Model file for the job. Use its own axes, mm. A direction names the side the tool comes from. Round coordinates to 2 decimals unless told otherwise and drop trailing zeros. Loops run counter-clockwise (first coordinate to the right, second up) from the corner with the lowest first, then second, coordinate; pieces in that order, holes last. Notation, with made-up numbers: M 6,-7.75 L 48,-7.75 A18 cw 48,-3.75 Z; hole C 30.5,-24 d10. An arc over 180 degrees is marked long. Use a Markdown table: item, result. Add a question column.
Item 1: Two-plate mould, pull along Y, no slides. Class faces 4 (the flat face through (8, -1, 3.6)), 5 (the cylindrical face through (-2.8, 0.1, 3.8)), 6 (the cylindrical face through (-2.15, 0.09, 3.69)): +Y half, -Y half, draft (parallel to the pull), parting line (faces both ways), or undercut.
Item 2: Saw through at C-C on z = 3.1. Write the cut outline in (x, y) (3 decimals), then the cut area to 3 significant figures.
Item 3: Wall check: L1, parallel to Y at x = 0, z = 3.1 (3 decimals); L2, parallel to Z at x = 3.5, y = 2.55; L3, parallel to Z at x = -0.75, y = -0.25. Give the ranges that are in metal, low to high. Write a range as from..to.
Item 4: Saw through at B-B on x = 11. Write the cut outline in (y, z).
Item 5: Saw through at D-D on x = 8. Write the cut outline in (y, z).
Item 6: Pin check, flat tips, straight feed: P1, Ø2, axis at y = 0.5, z = 1, coming from the -X side; P2, Ø2, axis at x = 0, y = 0, coming from the -Z side; P3, Ø2, axis at x = 0, y = 0.5, coming from the +Z side; P4, Ø1.5, axis at x = 9.5, z = 2.5, coming from the +Y side. Stop position of each tip, or through.
Item 7: Tool access for faces 1 (the cylindrical face through (-3, 0, 1)), 2 (the flat face through (-1, 0, 3.3)), 3 (the cylindrical face through (4.6, -0.3, 2.6)): list every direction of +Z, -Z, +X, -X, +Y, -Y with a clear straight run to the whole face (end or side of a thin tool).
```python
from build123d import *

# Parameters (mm, degrees)
SKETCH2_R           = 3
SKETCH2_R_2         = 2.8
BOSS_EXTRUDE1_DEPTH = 3.6
SKETCH2_3_R         = 2.8
SKETCH2_3_R_2       = 2.15
BOSS_EXTRUDE2_DEPTH = 4.1
BOSS_EXTRUDE3_START = 2.7
SKETCH2_4_R         = 2.15
SKETCH2_4_R_2       = 0.625
BOSS_EXTRUDE3_DEPTH = 0.6
SKETCH2_5_R         = 2.15
BOSS_EXTRUDE4_DEPTH = 2.7
BOSS_EXTRUDE5_START = 3.6
SKETCH2_6_R         = 0.5
BOSS_EXTRUDE5_DEPTH = 2


with BuildPart() as part:
    # Sketch2 → Boss-Extrude1 (new body)
    with BuildSketch(Plane.XY):
        Circle(SKETCH2_R)
        Circle(SKETCH2_R_2, mode=Mode.SUBTRACT)
    extrude(amount=BOSS_EXTRUDE1_DEPTH)

    # Sketch2<3> → Boss-Extrude2 (add)
    with BuildSketch(Plane.XY):
        Circle(SKETCH2_3_R)
        Circle(SKETCH2_3_R_2, mode=Mode.SUBTRACT)
    extrude(amount=BOSS_EXTRUDE2_DEPTH)

    # Sketch2<4> → Boss-Extrude3 (add)
    with BuildSketch(Plane.XY.offset(BOSS_EXTRUDE3_START)):
        Circle(SKETCH2_4_R)
        Circle(SKETCH2_4_R_2, mode=Mode.SUBTRACT)
    extrude(amount=BOSS_EXTRUDE3_DEPTH)

    # Sketch2<5> → Boss-Extrude4 (add)
    with BuildSketch(Plane.XY):
        Circle(SKETCH2_5_R)
        Polygon((-0.374241043, 1.760665681), (0, 2), (0.374241043, 1.760665681), (0.813473286, 1.827090915), (1.058013454, 1.45623059), (1.486289651, 1.338261213), (1.558845727, 0.9), (1.902113033, 0.618033989), (1.790139412, 0.188151234), (1.989043791, -0.209056927), (1.711901729, -0.55623059), (1.732050808, -1), (1.337660686, -1.204435091), (1.175570505, -1.618033989), (0.732125958, -1.644381824), (0.415823382, -1.956295201), (0, -1.8), (-0.415823382, -1.956295201), (-0.732125958, -1.644381824), (-1.175570505, -1.618033989), (-1.337660686, -1.204435091), (-1.732050808, -1), (-1.711901729, -0.55623059), (-1.989043791, -0.209056927), (-1.790139412, 0.188151234), (-1.902113033, 0.618033989), (-1.558845727, 0.9), (-1.486289651, 1.338261213), (-1.058013454, 1.45623059), (-0.813473286, 1.827090915), align=None, mode=Mode.SUBTRACT)
    extrude(amount=BOSS_EXTRUDE4_DEPTH)

    # Sketch2<6> → Boss-Extrude5 (add)
    with BuildSketch(Plane.XY.offset(BOSS_EXTRUDE5_START)):
        with BuildLine():
            Line((14.142857143, 1.994891435), (0.214285714, 2.992337152))
            ThreePointArc((0.214285714, 2.992337152), (3, 0), (0.214285714, -2.992337152))
            Line((0.214285714, -2.992337152), (14.142857143, -1.994891435))
            ThreePointArc((14.142857143, -1.994891435), (16, 0), (14.142857143, 1.994891435))
        make_face()
        with Locations((5, 0)):
            Circle(SKETCH2_6_R, mode=Mode.SUBTRACT)
        with Locations((8, 0)):
            Circle(SKETCH2_6_R, mode=Mode.SUBTRACT)
        with Locations((11, 0)):
            Circle(SKETCH2_6_R, mode=Mode.SUBTRACT)
        with Locations((14, 0)):
            Circle(SKETCH2_6_R, mode=Mode.SUBTRACT)
    extrude(amount=-BOSS_EXTRUDE5_DEPTH)


solid = part.part
```
Entries:
| question | item | result |
|---|---|---|
| 1 | face 4 | draft |
| 1 | face 5 | parting line |
| 1 | face 6 | undercut |
| 2 | outline | M 0.214,-2.992 L 14.143,-1.995 A2 ccw 14.143,1.995 L 0.214,2.992 A3 ccw long Z; hole C 0,0 d1.25; hole C 5,0 d1; hole C 8,0 d1; hole C 11,0 d1; hole C 14,0 d1 |
| 2 | area | 86.2 mm2 |
| 3 | L1 | -3..-0.625, 0.625..3 |
| 3 | L2 | 1.6..3.6 |
| 3 | L3 | 2.7..3.3 |
| 4 | outline | M -2.22,1.6 L -0.5,1.6 L -0.5,3.6 L -2.22,3.6 Z; M 0.5,1.6 L 2.22,1.6 L 2.22,3.6 L 0.5,3.6 Z |
| 5 | outline | M -2.43,1.6 L -0.5,1.6 L -0.5,3.6 L -2.43,3.6 Z; M 0.5,1.6 L 2.43,1.6 L 2.43,3.6 L 0.5,3.6 Z |
| 6 | P1 | x = -3 |
| 6 | P2 | z = 2.7 |
| 6 | P3 | z = 3.3 |
| 6 | P4 | y = 2.38 |
| 7 | face 1 | -Z |
| 7 | face 2 | +Z |
| 7 | face 3 | +Z, -Z |
